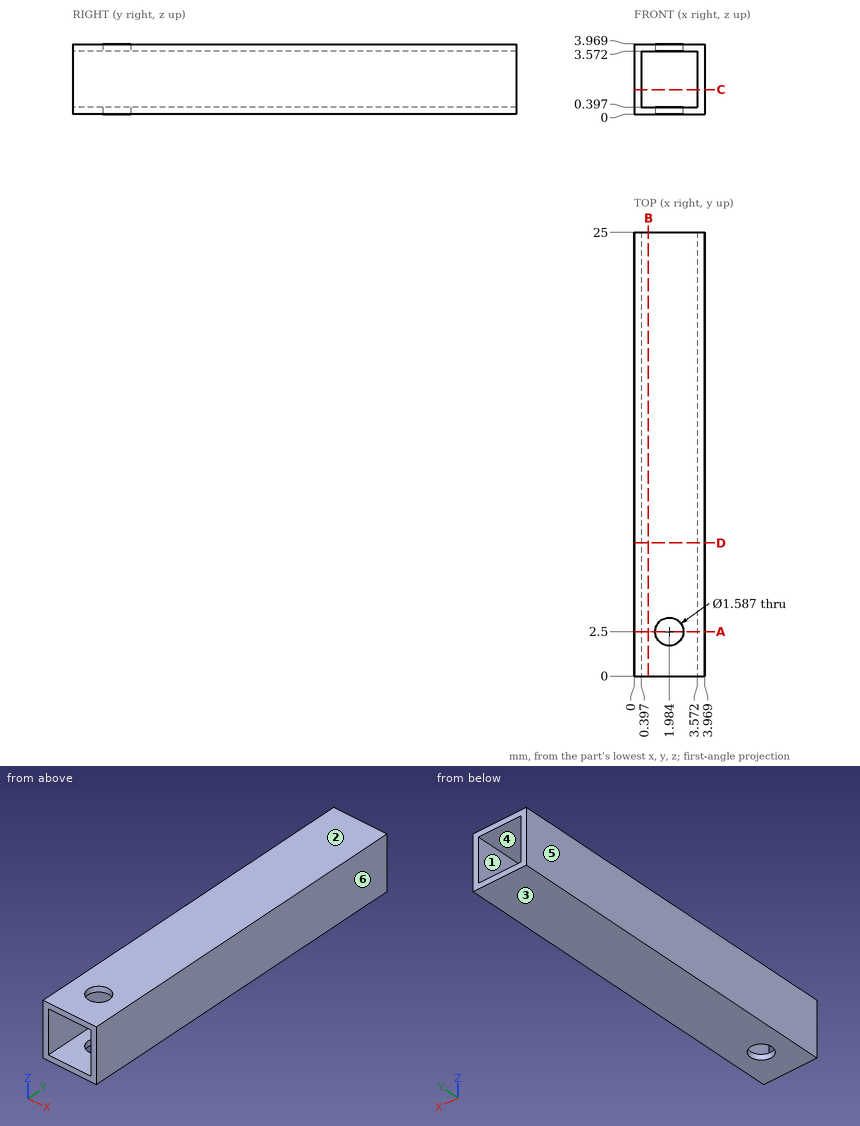
Verification items for this drawing (mm, ordinates from the low corner). A direction names the side the tool comes from. Give positions to 0.01 mm unless a question says otherwise; leave off trailing zeros. Loops run counter-clockwise (first coordinate to the right, second up) from the corner with the lowest first, then second, coordinate; pieces in that order, holes last.
1. Release check for a two-part mould opening along X. For the marked faces 3, 4, 5 and 6 record: +X half, -X half, draft (parallel to the pull), parting line (faces both ways), or undercut.
Derived:
face 3: draft
face 4: undercut
face 5: -X half
face 6: +X half
2. Material ranges on probe 1 along Z at (x, y) = (2.6, 1.5); probe 2 along X at (y, z) = (2.5, 3.75), recorded low to high.
Derived:
probe 1: z = 0 to 0.4, 3.57 to 3.97
probe 2: x = 0 to 1.19, 2.78 to 3.97
3. Cross-section at D-D on y = 7.5. Record the cut outline in (x, z).
Derived:
outline: (0, 0) - (3.97, 0) - (3.97, 3.97) - (0, 3.97) - close; hole (0.4, 0.4) - (3.57, 0.4) - (3.57, 3.57) - (0.4, 3.57) - close
4. Cross-section at C-C on z = 1.4. Record the cut outline in (x, y).
Derived:
outline: (0, 0) - (0.4, 0) - (0.4, 25) - (0, 25) - close; (3.57, 0) - (3.97, 0) - (3.97, 25) - (3.57, 25) - close
5. Cross-section at A-A on y = 2.5. Record the cut outline in (x, z).
Derived:
outline: (0, 0) - (1.19, 0) - (1.19, 0.4) - (0.4, 0.4) - (0.4, 3.57) - (1.19, 3.57) - (1.19, 3.97) - (0, 3.97) - close; (2.78, 0) - (3.97, 0) - (3.97, 3.97) - (2.78, 3.97) - (2.78, 3.57) - (3.57, 3.57) - (3.57, 0.4) - (2.78, 0.4) - close
6. Go/stop test with a flat-tipped pin: P1, Ø1, axis at x = 1.98, y = 2.5, coming from the -Z side. Record where the tip stops, or that it passes through.
Derived:
P1: passes through
7. Cross-section at B-B on x = 0.8. Record the cut outline in (y, z).
Derived:
outline: (0, 0) - (25, 0) - (25, 0.4) - (0, 0.4) - close; (0, 3.57) - (25, 3.57) - (25, 3.97) - (0, 3.97) - close
8. Tool access check on the marked faces 1 and 2. Record the directions out of +Z, -Z, +X, -X, +Y, -Y that give a thin tool (end or side, any length) a straight path to the whole face; none if there is none.
Derived:
face 1: +Y, -Y
face 2: +Z, +X, -X, +Y, -Y
